from build123d import *

# Parameters (mm, degrees)
SKETCH1_W           = 50
SKETCH1_H           = 8
SKETCH1_R           = 1.5
BOSS_EXTRUDE1_DEPTH = 3
SKETCH2_W           = 3
SKETCH2_H           = 8
BOSS_EXTRUDE2_DEPTH = 20
SKETCH3_W           = 8
SKETCH3_H           = 8
SKETCH3_R           = 1.5
BOSS_EXTRUDE3_DEPTH = 3


with BuildPart() as part:
    # Sketch1 → Boss-Extrude1 (new body)
    with BuildSketch(Plane(origin=(0, 0, 0), x_dir=(1, 0, 0), z_dir=(0, 1, 0))):
        Rectangle(SKETCH1_W, SKETCH1_H)
        with Locations(Location((-13.25, 0, 0), (0, 0, 270))):
            Circle(SKETCH1_R, mode=Mode.SUBTRACT)
        with Locations(Location((13.25, 0, 0), (0, 0, 270))):
            Circle(SKETCH1_R, mode=Mode.SUBTRACT)
    extrude(amount=BOSS_EXTRUDE1_DEPTH)

    # Sketch2 → Boss-Extrude2 (add)
    with BuildSketch(Plane.XZ):
        with Locations((-23.5, 0)):
            Rectangle(SKETCH2_W, SKETCH2_H)
    boss_extrude2 = extrude(amount=BOSS_EXTRUDE2_DEPTH)

    # Sketch3 → Boss-Extrude3 (add)
    with BuildSketch(Plane(origin=(0, -20, 0), x_dir=(-1, 0, 0), z_dir=(0, -1, 0))):
        with Locations((29, 0)):
            Rectangle(SKETCH3_W, SKETCH3_H)
        with Locations(Location((29, 0, 0), (0, 0, 90))):
            Circle(SKETCH3_R, mode=Mode.SUBTRACT)
    boss_extrude3 = extrude(amount=-BOSS_EXTRUDE3_DEPTH)

    # Mirror1: Boss-Extrude2, Boss-Extrude3 across plane
    add(boss_extrude2.mirror(Plane(origin=(0, 0, 0), x_dir=(0, 0, 1), z_dir=(1, 0, 0))))
    add(boss_extrude3.mirror(Plane(origin=(0, 0, 0), x_dir=(0, 0, 1), z_dir=(1, 0, 0))))


solid = part.part
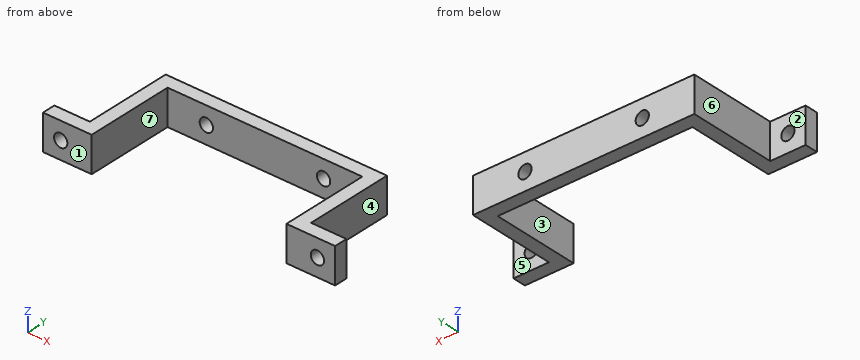
Could you check a few things on this model? Use its own coordinates, in mm. Face numbers are marked on the shaded views. A direction names the side the tool comes from. Coordinates: 2 decimals unless noted, no trailing zeros. Order: outer loops, then holes, each group sorted by start corner. A loop starts at its lowest first (then second) coordinate and runs counter-clockwise, first axis right, second up.
Q1. Suppose I cut it at C-C on z = -2.5. Please give me the cut outline in (x, y).
Q2. Which directions (+Z, -Z, +X, -X, +Y, -Y) give clear straight access to the entire face, cutting with the end or side of a thin tool? Please do the marked faces 1, 2 and 3.
Q3. Please list where these lines run through material, in increasing order: L1, parallel to X at y = -18.9, z = 0; L2, parallel to X at y = -6.5, z = 0.75; L3, parallel to X at y = 1.7, z = 0.
Q4. Suppose I cut it at D-D on x = -17.5. Please give me the cut outline in (y, z), and give its area (3 significant figures).
Q5. Will these pins go through, and if not, where does the flat tip stop? pin 1 (2.5 mm diameter, centred on x = 30, z = -0.5, fed in from +Y); pin 2 (4 mm diameter, centred on y = -9, z = 3, fed in from -X); pin 3 (2.5 mm diameter, centred on y = -3.5, z = 1, fed in from +X).
Q6. Thinking about a two-plate mould opening in X: for the marked faces 4, 5, 6 and 7, which applies, released by +X, released by -X, zero draft, split by the parting line, or undercut?
Q7. Suppose I cut it at A-A on z = 0. Please give me the cut outline in (x, y), and give its area (3 significant figures).
Q8. Suppose I cut it at B-B on x = 13.25. Please give me the cut outline in (y, z), and give its area (3 significant figures).
Answer:
1. outline: (-33, -20) - (-22, -20) - (-22, 0) - (22, 0) - (22, -20) - (33, -20) - (33, -17) - (25, -17) - (25, 3) - (-25, 3) - (-25, -17) - (-33, -17) - close
2. face 1: +Z, -Z, +X, -X, -Y
2. face 2: +Z, -Z, -X, +Y
2. face 3: +Z, -Z, -Y
3. L1: x = -33 to -30.5, -27.5 to -22, 22 to 27.5, 30.5 to 33
3. L2: x = -25 to -22, 22 to 25
3. L3: x = -25 to -14.75, -11.75 to 11.75, 14.75 to 25
4. outline: (0, -4) - (3, -4) - (3, 4) - (0, 4) - close
4. area: 24.0 mm2
5. pin 1: stops at y = -17
5. pin 2: stops at x = -25
5. pin 3: stops at x = 25
6. face 4: released by +X
6. face 5: zero draft
6. face 6: released by -X
6. face 7: undercut
7. outline: (-33, -20) - (-30.5, -20) - (-30.5, -17) - (-33, -17) - close; (-27.5, -20) - (-22, -20) - (-22, 0) - (-14.75, 0) - (-14.75, 3) - (-25, 3) - (-25, -17) - (-27.5, -17) - close; (-11.75, 0) - (11.75, 0) - (11.75, 3) - (-11.75, 3) - close; (14.75, 0) - (22, 0) - (22, -20) - (27.5, -20) - (27.5, -17) - (25, -17) - (25, 3) - (14.75, 3) - close; (30.5, -20) - (33, -20) - (33, -17) - (30.5, -17) - close
7. area: 282 mm2
8. outline: (0, -4) - (3, -4) - (3, -1.5) - (0, -1.5) - close; (0, 1.5) - (3, 1.5) - (3, 4) - (0, 4) - close
8. area: 15.0 mm2
